Design review of the part built by this model. Coordinates are the model's own, in mm. A direction names the side the tool comes from. Round coordinates to 2 decimals unless told otherwise and drop trailing zeros. Loops run counter-clockwise (first coordinate to the right, second up) from the corner with the lowest first, then second, coordinate; pieces in that order, holes last. Notation, with made-up numbers: (42.5, 75.25) -> (80.5, 75.25) arc R24 ccw to (80.5, 96.25) -> close; hole circle Ø3 at (-31.75, -40). An arc over 180 degrees is marked (long way). Answer as CSV lines item,"result". Start each with the question number.
(1) Draft analysis for pull direction Y (two halves, no side actions). For faces 4 (the face through (34, -37, 0)), 5 (the face through (0, 37, 0)), 6 (the face through (35.886, 37.25, 27.313)), 7 (the face through (-27.69, -38.47, 16.1)), state which applies: +Y half, -Y half, draft (parallel to the pull), parting line (faces both ways), or undercut.
(2) Machinability: for faces 1 (the face through (-38.75, -13.95, 22.75)), 2 (the face through (-31, 5, -5)), 3 (the face through (-34, 0, 29)), which of the approach directions +Z, -Z, +X, -X, +Y, -Y give a long, thin tool a straight path to every point of the face, cutting with its end or side? Answer none if there is none.
(3) Take a section at C-C, the plane z = 10. Write out the cut boundary in (x, y).
(4) Take a section at A-A, the plane x = -3. Write out the cut boundary in (y, z).
(5) For P1, Ø3, axis at y = -20, z = -8.5, coming from the +X side; P2, Ø6, axis at y = -8.5, z = -6, coming from the -X side; P3, Ø3.5, axis at y = 14.62, z = 19.75, coming from the +X side, all flat-tipped, find the tip position at first contact; note any pin that passes through.
(6) To check wall thickness, follow line 1 (X direction, y = -14.5, z = 1); line 2 (Y direction, x = -1.5, z = 26); line 3 (X direction, y = 13.5, z = 17). State the ranges of each line that lie inside material, in increasing order. Write a range as from..to.
from build123d import *

# Parameters (mm, degrees)
BOSS_EXTRUDE1_DEPTH     = 31.75
SHELL1_T                = -6
FILLET1_R               = 5.334
CUT_EXTRUDE1_DEPTH      = 1.2954
FILLET2_R               = 0.254
FILLET3_R               = 0.127
BOSS_EXTRUDE2_DEPTH     = 31.75
SKETCH4_R               = 3.025
CUT_EXTRUDE2_DEPTH      = 9
MIRROR2_COPY_1_DEPTH    = 31.75
MIRROR2_COPY_2_SKETCH_R = 3.025
MIRROR2_COPY_2_DEPTH    = 9
SKETCH8_W               = 12
SKETCH8_H               = 58.443650814
BOSS_EXTRUDE3_DEPTH     = 6
SKETCH12_R              = 3.025
CUT_EXTRUDE6_DEPTH      = 2.54
SKETCH13_R              = 6.35
CUT_EXTRUDE10_DEPTH     = 6
SKETCH16_R              = 11.43
CUT_EXTRUDE14_DEPTH     = 3


with BuildPart() as part:
    # Sketch1 → Boss-Extrude1 (new, symmetric)
    with BuildSketch(Plane.XY):
        Polygon((-34, -37), (-34, -16.68), (-34, 16.68), (-34, 37), (34, 37), (34, -37), align=None)
    extrude(amount=BOSS_EXTRUDE1_DEPTH, both=True)

    # Shell1
    shell1_openings = [part.faces().sort_by_distance(p)[0] for p in [
        (0, 0, 31.75),
    ]]
    offset(amount=SHELL1_T, openings=shell1_openings, kind=Kind.INTERSECTION)

    # Fillet1
    fillet1_edges = [part.edges().sort_by_distance(p)[0] for p in [
        (-34, -37, 0),
        (-34, 37, 0),
        (34, 37, 0),
        (34, -37, 0),
        (-28, -31, 3),
        (28, -31, 3),
        (28, 31, 3),
        (-28, 31, 3),
    ]]
    fillet(fillet1_edges, radius=FILLET1_R)

    # Sketch2 → Cut-Extrude1 (cut)
    with BuildSketch(Plane.XY.offset(31.75)):
        with BuildLine():
            Line((32.2827, -25.666), (32.2827, 25.666))
            ThreePointArc((32.2827, 25.666), (29.466033783, 32.466033783), (22.666, 35.2827))
            Line((22.666, 35.2827), (-22.666, 35.2827))
            ThreePointArc((-22.666, 35.2827), (-29.466033783, 32.466033783), (-32.2827, 25.666))
            Line((-32.2827, 25.666), (-32.2827, -25.666))
            ThreePointArc((-32.2827, -25.666), (-29.466033783, -32.466033783), (-22.666, -35.2827))
            Line((-22.666, -35.2827), (22.666, -35.2827))
            ThreePointArc((22.666, -35.2827), (29.466033783, -32.466033783), (32.2827, -25.666))
        make_face()
        with BuildLine():
            Line((-29.7173, 25.666), (-29.7173, -25.666))
            ThreePointArc((-29.7173, -25.666), (-27.652022046, -30.652022046), (-22.666, -32.7173))
            Line((-22.666, -32.7173), (22.666, -32.7173))
            ThreePointArc((22.666, -32.7173), (27.652022046, -30.652022046), (29.7173, -25.666))
            Line((29.7173, -25.666), (29.7173, 25.666))
            ThreePointArc((29.7173, 25.666), (27.652022046, 30.652022046), (22.666, 32.7173))
            Line((22.666, 32.7173), (-22.666, 32.7173))
            ThreePointArc((-22.666, 32.7173), (-27.652022046, 30.652022046), (-29.7173, 25.666))
        make_face(mode=Mode.SUBTRACT)
    extrude(amount=-CUT_EXTRUDE1_DEPTH, mode=Mode.SUBTRACT)

    # Fillet2
    fillet2_edges = [part.edges().sort_by_distance(p)[0] for p in [
        (29.466033783, -32.466033783, 30.4546),
        (0, -35.2827, 30.4546),
        (-29.466033783, -32.466033783, 30.4546),
        (-32.2827, 0, 30.4546),
        (-29.466033783, 32.466033783, 30.4546),
        (0, 35.2827, 30.4546),
        (29.466033783, 32.466033783, 30.4546),
        (32.2827, 0, 30.4546),
        (0, 32.7173, 30.4546),
        (-27.652022046, 30.652022046, 30.4546),
        (-29.7173, 0, 30.4546),
        (-27.652022046, -30.652022046, 30.4546),
        (0, -32.7173, 30.4546),
        (27.652022046, -30.652022046, 30.4546),
        (29.7173, 0, 30.4546),
        (27.652022046, 30.652022046, 30.4546),
    ]]
    fillet(fillet2_edges, radius=FILLET2_R)

    # Fillet3
    fillet3_edges = [part.edges().sort_by_distance(p)[0] for p in [
        (29.466033783, -32.466033783, 31.75),
        (32.2827, 0, 31.75),
        (29.466033783, 32.466033783, 31.75),
        (0, 35.2827, 31.75),
        (-29.466033783, 32.466033783, 31.75),
        (-32.2827, 0, 31.75),
        (-29.466033783, -32.466033783, 31.75),
        (0, -35.2827, 31.75),
        (-27.652022046, 30.652022046, 31.75),
        (0, 32.7173, 31.75),
        (27.652022046, 30.652022046, 31.75),
        (29.7173, 0, 31.75),
        (27.652022046, -30.652022046, 31.75),
        (0, -32.7173, 31.75),
        (-27.652022046, -30.652022046, 31.75),
        (-29.7173, 0, 31.75),
    ]]
    fillet(fillet3_edges, radius=FILLET3_R)

    # Sketch3 → Boss-Extrude2 (add)
    with BuildSketch(Plane.XY.offset(31.75)):
        with BuildLine():
            Line((34, -29.221825407), (34, -31.666))
            ThreePointArc((34, -31.666), (32.437707571, -35.437707571), (28.666, -37))
            Line((28.666, -37), (26.221825407, -37))
            Line((26.221825407, -37), (29.202282953, -39.980457546))
            ThreePointArc((29.202282953, -39.980457546), (36.980457546, -39.980457546), (36.980457546, -32.202282953))
            Line((36.980457546, -32.202282953), (34, -29.221825407))
        make_face()
    boss_extrude2 = extrude(amount=-BOSS_EXTRUDE2_DEPTH)

    # Sketch4 → Cut-Extrude2 (cut)
    with BuildSketch(Plane.XY.offset(31.75)):
        with Locations((33.09137025, -36.09137025)):
            Circle(SKETCH4_R)
    cut_extrude2 = extrude(amount=-CUT_EXTRUDE2_DEPTH, mode=Mode.SUBTRACT)

    # Mirror1: Boss-Extrude2, Cut-Extrude2 across plane
    add(boss_extrude2.mirror(Plane.ZX))
    add(cut_extrude2.mirror(Plane.ZX), mode=Mode.SUBTRACT)

    # Mirror2: Boss-Extrude2, Cut-Extrude2 across plane
    add(boss_extrude2.mirror(Plane(origin=(0, 0, 0), x_dir=(0, 0, 1), z_dir=(1, 0, 0))))
    add(cut_extrude2.mirror(Plane(origin=(0, 0, 0), x_dir=(0, 0, 1), z_dir=(1, 0, 0))), mode=Mode.SUBTRACT)

    # Mirror2 copy 1 sketch → Mirror2 copy 1 (add)
    with BuildSketch(Plane(origin=(0, 0, 31.75), x_dir=(-1, 0, 0), z_dir=(0, 0, 1))):
        with BuildLine():
            Line((34, -29.221825407), (34, -31.666))
            ThreePointArc((34, -31.666), (32.437707571, -35.437707571), (28.666, -37))
            Line((28.666, -37), (26.221825407, -37))
            Line((26.221825407, -37), (29.202282953, -39.980457546))
            ThreePointArc((29.202282953, -39.980457546), (36.980457546, -39.980457546), (36.980457546, -32.202282953))
            Line((36.980457546, -32.202282953), (34, -29.221825407))
        make_face()
    extrude(amount=-MIRROR2_COPY_1_DEPTH)

    # Mirror2 copy 2 sketch → Mirror2 copy 2 (cut)
    with BuildSketch(Plane(origin=(0, 0, 31.75), x_dir=(-1, 0, 0), z_dir=(0, 0, 1))):
        with Locations((33.09137025, -36.09137025)):
            Circle(MIRROR2_COPY_2_SKETCH_R)
    extrude(amount=-MIRROR2_COPY_2_DEPTH, mode=Mode.SUBTRACT)

    # Sketch8 → Boss-Extrude3 (add)
    with BuildSketch(Plane.ZY.offset(34)):
        with Locations((19.75, 0)):
            Rectangle(SKETCH8_W, SKETCH8_H)
    boss_extrude3 = extrude(amount=BOSS_EXTRUDE3_DEPTH)

    # Sketch12 → Cut-Extrude6 (cut)
    with BuildSketch(Plane.ZY.offset(40)):
        with Locations(Location((19.75, 14.616825407, 0), (0, 0, 270))):
            Circle(SKETCH12_R)
        with Locations(Location((19.75, -14.339174593, 0), (0, 0, 270))):
            Circle(SKETCH12_R)
    cut_extrude6 = extrude(amount=-CUT_EXTRUDE6_DEPTH, mode=Mode.SUBTRACT)

    # Sketch13 → Cut-Extrude10 (cut)
    with BuildSketch(Plane.ZY.offset(34)):
        with Locations(Location((0, 0, 0), (0, 0, 270))):
            Circle(SKETCH13_R)
    extrude(amount=-CUT_EXTRUDE10_DEPTH, mode=Mode.SUBTRACT)

    # Sketch16 → Cut-Extrude14 (cut)
    with BuildSketch(Plane(origin=(-28, 0, 0), x_dir=(0, 0, -1), z_dir=(1, 0, 0))):
        with Locations(Location((0, 0, 0), (0, 0, 90))):
            Circle(SKETCH16_R)
    extrude(amount=-CUT_EXTRUDE14_DEPTH, mode=Mode.SUBTRACT)

    # Mirror5: Boss-Extrude3 across plane
    add(boss_extrude3.mirror(Plane(origin=(0, 0, 0), x_dir=(0, 0, 1), z_dir=(1, 0, 0))))

    # Mirror6: Cut-Extrude6 across plane
    add(cut_extrude6.mirror(Plane(origin=(0, 0, 0), x_dir=(0, 0, 1), z_dir=(1, 0, 0))), mode=Mode.SUBTRACT)


solid = part.part
The answers:
1,face 4,"draft"
1,face 5,"+Y half"
1,face 6,"undercut"
1,face 7,"-Y half"
2,face 1,"-X"
2,face 2,"none"
2,face 3,"+Z, -X"
3,outline,"(-36.98, -32.2) arc R5.5 ccw to (-29.2, -39.98) -> (-26.22, -37) -> (26.22, -37) -> (29.2, -39.98) arc R5.5 ccw to (36.98, -32.2) -> (34, -29.22) -> (34, 29.22) -> (36.98, 32.2) arc R5.5 ccw to (29.2, 39.98) -> (26.22, 37) -> (-26.22, 37) -> (-29.2, 39.98) arc R5.5 ccw to (-36.98, 32.2) -> (-34, 29.22) -> (-34, -29.22) -> close; hole (-31, -5.54) -> (-28, -5.54) -> (-28, -25.67) arc R5.33 ccw to (-22.67, -31) -> (22.67, -31) arc R5.33 ccw to (28, -25.67) -> (28, 25.67) arc R5.33 ccw to (22.67, 31) -> (-22.67, 31) arc R5.33 ccw to (-28, 25.67) -> (-28, 5.54) -> (-31, 5.54) -> close"
4,outline,"(-37, -31.75) -> (37, -31.75) -> (37, 31.75) -> (35.41, 31.75) arc R0.13 ccw to (35.28, 31.62) -> (35.28, 30.71) arc R0.25 cw to (35.03, 30.45) -> (32.97, 30.45) arc R0.25 cw to (32.72, 30.71) -> (32.72, 31.62) arc R0.13 ccw to (32.59, 31.75) -> (31, 31.75) -> (31, -25.75) -> (-31, -25.75) -> (-31, 31.75) -> (-32.59, 31.75) arc R0.13 ccw to (-32.72, 31.62) -> (-32.72, 30.71) arc R0.25 cw to (-32.97, 30.45) -> (-35.03, 30.45) arc R0.25 cw to (-35.28, 30.71) -> (-35.28, 31.62) arc R0.13 ccw to (-35.41, 31.75) -> (-37, 31.75) -> close"
5,P1,"x = 34"
5,P2,"x = -34"
5,P3,"x = 37.46"
6,line 1,"-34..-28, 28..34"
6,line 2,"-37..-31, 31..37"
6,line 3,"-37.46..-28, 28..37.46"
